```python
from build123d import *

# Parameters (mm, degrees)
F1_DEPTH = 304.8


with BuildPart() as f1:
    # F0 (on Top) → F1 (new body)
    with BuildSketch(Plane.XY):
        Polygon((-44.45, 19.05), (-44.45, 0), (-36.83, 0), (-36.83, 11.43), (36.83, 11.43), (36.83, 0), (44.45, 0), (44.45, 19.05), align=None)
    extrude(amount=F1_DEPTH)

    # F2: F1 across plane


with BuildPart() as f1_1:
    add(f1.part)
    add(f1.part.mirror(Plane.XZ))


solid = f1_1.part
```
Work out the finished part from the listing and answer in its coordinate system (mm). A direction names the side the tool comes from. Give positions to 0.01 mm unless a question says otherwise; leave off trailing zeros. Write each loop counter-clockwise with the first axis right and the second up, starting at its lowest first coordinate (ties: lowest second). Pieces come first, ordered by that corner, then holes. Notation, with made-up numbers: (-35.75, 43.25) -> (-9.75, 43.25) arc R23 cw to (-9.75, 60.25) -> close; hole circle Ø7 at (-39, 83.5). An arc over 180 degrees is marked (long way). Write item = value, one per line.
Q1. A tool of negligible diameter and unlimited length cuts with its end or side. For faces 4 (the flat face through (36.83, 0, 150)), 5 (the flat face through (44.45, 0, 150)), from which of +Z, -Z, +X, -X, +Y, -Y can it reach the whole face along a straight path? Write none if from no direction.
Computed values:
face_4 = +Z, -Z
face_5 = +Z, -Z, +X, +Y, -Y
Q2. Section C-C on x = -16.5 is taken. Determine the outline of the cut face in (y, z), and give its area (3 significant figures).
Computed values:
outline = (-19.05, 0) -> (-11.43, 0) -> (-11.43, 304.8) -> (-19.05, 304.8) -> close; (11.43, 0) -> (19.05, 0) -> (19.05, 304.8) -> (11.43, 304.8) -> close
area = 4,650 mm^2
Q3. Consider line 1 along X through (y, z) = (-1, 207); line 2 along Y through (x, z) = (-22.5, 43). Determine where each line is inside the solid, lowest interval first.
Computed values:
line_1 = -44.45 to -36.83, 36.83 to 44.45
line_2 = -19.05 to -11.43, 11.43 to 19.05
Q4. For a pull along X with two mould halves and no side action, classify faces 1 (the flat face through (1, 19.05, 150)), 2 (the flat face through (-44.45, 0, 150)), 3 (the flat face through (-1, -11.43, 150)) as pulls with the +X half, pulls with the -X half, needs draft (parallel to the pull), parting line crosses it, or undercut.
Computed values:
face_1 = needs draft
face_2 = pulls with the -X half
face_3 = undercut
Q5. Section B-B on y = 3 is taken. Determine the outline of the cut face in (x, z), and give its area (3 significant figures).
Computed values:
outline = (-44.45, 0) -> (-36.83, 0) -> (-36.83, 304.8) -> (-44.45, 304.8) -> close; (36.83, 0) -> (44.45, 0) -> (44.45, 304.8) -> (36.83, 304.8) -> close
area = 4,650 mm^2
Q6. Section A-A on z = 194 is taken. Determine the outline of the cut face in (x, y).
Computed values:
outline = (-44.45, -19.05) -> (44.45, -19.05) -> (44.45, 19.05) -> (-44.45, 19.05) -> close; hole (-36.83, -11.43) -> (36.83, -11.43) -> (36.83, 11.43) -> (-36.83, 11.43) -> close
